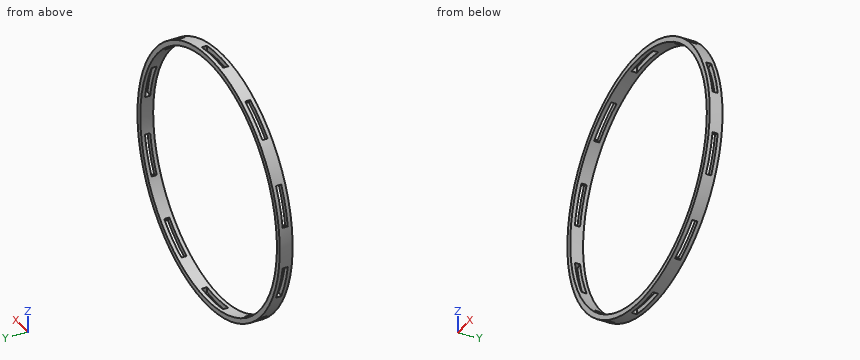
from build123d import *

# Parameters (mm, degrees)
SKETCH1_R           = 100
SKETCH1_R_2         = 96
BOSS_EXTRUDE1_DEPTH = 10
SKETCH2_W           = 30
SKETCH2_H           = 4
CUT_EXTRUDE1_DEPTH  = 101
CIRPATTERN1_COUNT   = 10


with BuildPart() as part:
    # Sketch1 → Boss-Extrude1 (new body)
    with BuildSketch(Plane(origin=(0, 0, 0), x_dir=(1, 0, 0), z_dir=(0, 1, 0))):
        Circle(SKETCH1_R)
        Circle(SKETCH1_R_2, mode=Mode.SUBTRACT)
    extrude(amount=BOSS_EXTRUDE1_DEPTH)

    # Sketch2 → Cut-Extrude1 (cut, through all)
    with BuildSketch(Plane.XY):
        with Locations((0, 5)):
            Rectangle(SKETCH2_W, SKETCH2_H)
    cut_extrude1 = extrude(amount=-CUT_EXTRUDE1_DEPTH, mode=Mode.SUBTRACT)

    # CirPattern1: Cut-Extrude1 ×10 about axis
    cirpattern1_axis = Axis((0, 0, 0), (0, 1, 0))
    for i in range(1, CIRPATTERN1_COUNT):
        add(cut_extrude1.rotate(cirpattern1_axis, i * 360 / CIRPATTERN1_COUNT), mode=Mode.SUBTRACT)


solid = part.part
Could you check a few things on this model? Use its own coordinates, in mm. Give positions to 0.01 mm unless a question says otherwise; leave off trailing zeros. Order: outer loops, then holes, each group sorted by start corner. A loop starts at its lowest first (then second) coordinate and runs counter-clockwise, first axis right, second up. Notation, with made-up numbers: (70.5, 55.25) - (117.5, 55.25) arc R26 cw to (117.5, 74.25) - close; hole circle Ø4 at (-17.5, 18). An arc over 180 degrees is marked (long way). Return JSON: item names as keys, results as strings. Group by question number.
Q1. Suppose I cut it at C-C, the plane z = 41. Please give me the cut outline in (x, y).
Q2. Suppose I cut it at B-B, the plane x = 0. Please give me the cut outline in (y, z).
Q3. Please list where these lines run through material, in increasing order: line 1 along X through (y, z) = (3, 0); line 2 along X through (y, z) = (8.5, -62); line 3 along Z through (x, y) = (-40, 6). Write a range as [from, to].
Q4. Suppose I cut it at D-D, the plane y = 8.5. Please give me the cut outline in (x, z).
Q5. Will these pins go through, and if not, where does the flat tip stop? pin 1 Ø1 at (y, z) = (5, 58.5) entering from -X; pin 2 Ø1.5 at (x, y) = (-2, 2) entering from -Z; pin 3 Ø1 at (x, y) = (-18.5, 7.5) entering from +Z.
Q6. Suppose I cut it at A-A, the plane z = 0. Please give me the cut outline in (x, y).
Resolved:
{
 "1": {"outline": "(-91.21, 0) - (-86.8, 0) - (-86.8, 3) - (-91.21, 3) - close; (-91.21, 7) - (-86.8, 7) - (-86.8, 10) - (-91.21, 10) - close; (86.8, 0) - (91.21, 0) - (91.21, 3) - (86.8, 3) - close; (86.8, 7) - (91.21, 7) - (91.21, 10) - (86.8, 10) - close"},
 "2": {"outline": "(0, -100) - (3, -100) - (3, -96) - (0, -96) - close; (0, 96) - (3, 96) - (3, 100) - (0, 100) - close; (7, -100) - (10, -100) - (10, -96) - (7, -96) - close; (7, 96) - (10, 96) - (10, 100) - (7, 100) - close"},
 "3": {"line 1": "x = [-100, -96], [96, 100]", "line 2": "x = [-78.46, -73.29], [73.29, 78.46]", "line 3": "z = [-91.65, -87.27], [87.27, 91.65]"},
 "4": {"outline": "circle Ø200 at (0, 0); hole circle Ø192 at (0, 0)"},
 "5": {"pin 1": "stops at x = -81.46", "pin 2": "stops at z = -99.99", "pin 3": "stops at z = 98.37"},
 "6": {"outline": "(-100, 0) - (-96, 0) - (-96, 10) - (-100, 10) - close; (96, 0) - (100, 0) - (100, 10) - (96, 10) - close"}
}
